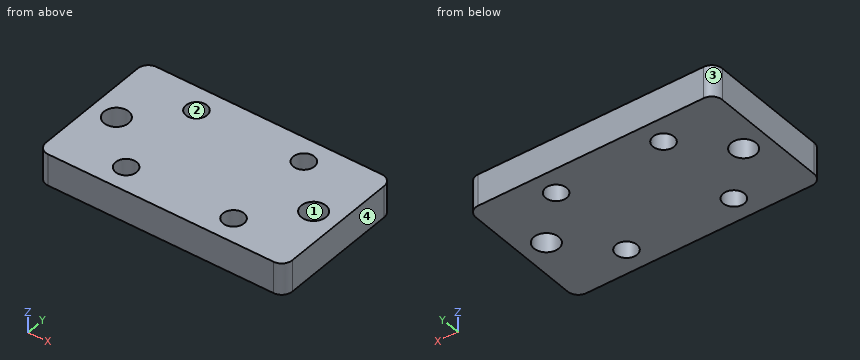
```python
from build123d import *

# Parameters (mm, degrees)
ESQUISSE1_W                  = 70
ESQUISSE1_H                  = 40
BOSS_EXTRU_1_DEPTH           = 9
ESQUISSE2_R                  = 3
ESQUISSE2_R_2                = 3.5
ENL_V_MAT_EXTRU_1_DEPTH      = 1
ENL_V_MAT_EXTRU_1_DEPTH_BACK = 10
CONG_1_R                     = 3


with BuildPart() as part:
    # Esquisse1 → Boss.-Extru.1 (new body)
    with BuildSketch(Plane.XY):
        with Locations((35, 20)):
            Rectangle(ESQUISSE1_W, ESQUISSE1_H)
    extrude(amount=BOSS_EXTRU_1_DEPTH)

    # Esquisse2 → Enlèv. mat.-Extru.1 (cut, two sides)
    with BuildSketch(Plane.XY.offset(9)) as enl_v_mat_extru_1_sk:
        with Locations((19.75, 33)):
            Circle(ESQUISSE2_R)
        with Locations((50.25, 33)):
            Circle(ESQUISSE2_R)
        with Locations((50.25, 7)):
            Circle(ESQUISSE2_R)
        with Locations((19.75, 7)):
            Circle(ESQUISSE2_R)
        with Locations((7, 20)):
            Circle(ESQUISSE2_R_2)
        with Locations((63, 20)):
            Circle(ESQUISSE2_R_2)
    extrude(amount=ENL_V_MAT_EXTRU_1_DEPTH, mode=Mode.SUBTRACT)
    extrude(enl_v_mat_extru_1_sk.sketch, amount=-ENL_V_MAT_EXTRU_1_DEPTH_BACK, mode=Mode.SUBTRACT)

    # Congé1
    cong_1_edges = [part.edges().sort_by_distance(p)[0] for p in [
        (0, 40, 4.5),
        (70, 40, 4.5),
        (70, 0, 4.5),
        (0, 0, 4.5),
    ]]
    fillet(cong_1_edges, radius=CONG_1_R)


solid = part.part
```
The listing builds one solid part. Answer for the finished solid, in the listing's coordinates (mm). Face numbers are marked on the shaded views. Coordinates: 2 decimals unless noted, no trailing zeros. Write each loop counter-clockwise with the first axis right and the second up, starting at its lowest first coordinate (ties: lowest second). Pieces come first, ordered by that corner, then holes. Notation, with made-up numbers: (1.25, 21.25) - (29.25, 21.25) arc R16 cw to (29.25, 48.25) - close; hole circle Ø10 at (-38.75, 18). An arc over 180 degrees is marked (long way). Return JSON: item names as keys, results as strings. Group by question number.
1. A cutting plane is placed at A-A, the plane y = 7. Determine the outline of the cut face in (x, z), plus the area to 3 significant figures.
2. A cutting plane is placed at D-D, the plane x = 50.25. Determine the outline of the cut face in (y, z), plus the area to 3 significant figures.
3. A cutting plane is placed at B-B, the plane x = 7. Determine the outline of the cut face in (y, z).
4. A cutting plane is placed at C-C, the plane z = 1.5. Determine the outline of the cut face in (x, y), plus the area to 3 significant figures.
5. Straight lines are drawn through the part: L1, parallel to Y at x = 7, z = 5; L2, parallel to Y at x = 19.75, z = 4; L3, parallel to X at y = 32, z = 6. For each, find the intervals that lie inside material, in ascending order.
6. Determine the mould class of the marked faces 1, 2, 3 and 4 for opening direction Y: released by +Y, released by -Y, zero draft, split by the parting line, or undercut.
Ans:
{
 "1": {"outline": "(0, 0) - (16.75, 0) - (16.75, 9) - (0, 9) - close; (22.75, 0) - (47.25, 0) - (47.25, 9) - (22.75, 9) - close; (53.25, 0) - (70, 0) - (70, 9) - (53.25, 9) - close", "area": "522 mm²"},
 "2": {"outline": "(0, 0) - (4, 0) - (4, 9) - (0, 9) - close; (10, 0) - (30, 0) - (30, 9) - (10, 9) - close; (36, 0) - (40, 0) - (40, 9) - (36, 9) - close", "area": "252 mm²"},
 "3": {"outline": "(0, 0) - (16.5, 0) - (16.5, 9) - (0, 9) - close; (23.5, 0) - (40, 0) - (40, 9) - (23.5, 9) - close"},
 "4": {"outline": "(0, 3) arc R3 ccw to (3, 0) - (67, 0) arc R3 ccw to (70, 3) - (70, 37) arc R3 ccw to (67, 40) - (3, 40) arc R3 ccw to (0, 37) - close; hole circle Ø7 at (7, 20); hole circle Ø6 at (19.75, 7); hole circle Ø6 at (19.75, 33); hole circle Ø6 at (50.25, 7); hole circle Ø6 at (50.25, 33); hole circle Ø7 at (63, 20)", "area": "2,600 mm²"},
 "5": {"L1": "0 to 16.5, 23.5 to 40", "L2": "0 to 4, 10 to 30, 36 to 40", "L3": "0 to 16.92, 22.58 to 47.42, 53.08 to 70"},
 "6": {"face 1": "undercut", "face 2": "undercut", "face 3": "released by +Y", "face 4": "zero draft"}
}
